Source: CAD feature listing. Evaluate the final solid. Frame: model axes, mm. Face numbers are marked on the shaded views. A direction names the side the tool comes from. Coordinates: 2 decimals unless noted, no trailing zeros. Loops run counter-clockwise (first coordinate to the right, second up) from the corner with the lowest first, then second, coordinate; pieces in that order, holes last. Notation, with made-up numbers: (-37.5, 0) -> (-3.5, 0) arc R9 ccw to (-3.5, 10) -> close; hole circle Ø1 at (-10, 31). An arc over 180 degrees is marked (long way). Answer as CSV lines item,"result".
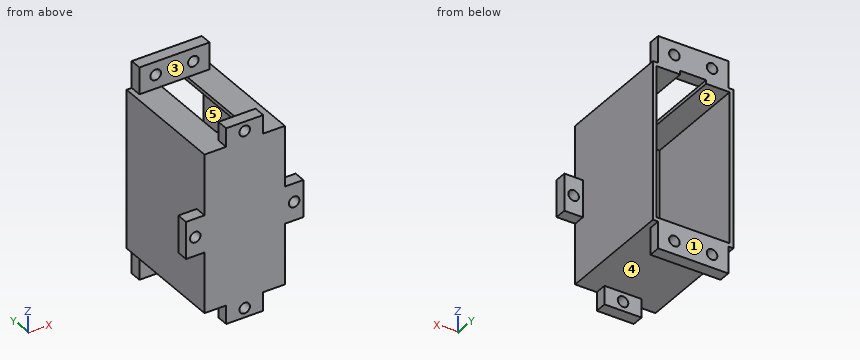
from build123d import *

# Parameters (mm, degrees)
SKETCH1_R           = 1.425
BOSS_EXTRUDE1_DEPTH = 3.175
SKETCH2_W           = 21.685
SKETCH2_H           = 42.7
SKETCH2_W_2         = 19.685
SKETCH2_H_2         = 40.7
BOSS_EXTRUDE2_DEPTH = 28.905
SKETCH3_W           = 18.923
SKETCH3_H           = 7.239
SKETCH3_R           = 1.425
BOSS_EXTRUDE3_DEPTH = 3.175
SKETCH4_W           = 7
SKETCH4_H           = 25.77275476
CUT_EXTRUDE1_DEPTH  = 3.175


with BuildPart() as part:
    # Sketch1 → Boss-Extrude1 (new body)
    with BuildSketch(Plane(origin=(0, 0, 0), x_dir=(1, 0, 0), z_dir=(0, 1, 0))):
        Polygon((10.8425, -21.35), (5, -21.35), (5, -26.35), (-5, -26.35), (-5, -21.35), (-10.8425, -21.35), (-10.8425, -5), (-15.8425, -5), (-15.8425, 5), (-10.8425, 5), (-10.8425, 21.35), (-5, 21.35), (-5, 26.35), (5, 26.35), (5, 21.35), (10.8425, 21.35), (10.8425, 5), (15.8425, 5), (15.8425, -5), (10.8425, -5), align=None)
        with Locations(Location((0, 23.85, 0), (0, 0, 270))):
            Circle(SKETCH1_R, mode=Mode.SUBTRACT)
        with Locations(Location((-13.3425, 0, 0), (0, 0, 270))):
            Circle(SKETCH1_R, mode=Mode.SUBTRACT)
        with Locations(Location((13.3425, 0, 0), (0, 0, 270))):
            Circle(SKETCH1_R, mode=Mode.SUBTRACT)
        with Locations(Location((0, -23.85, 0), (0, 0, 270))):
            Circle(SKETCH1_R, mode=Mode.SUBTRACT)
    extrude(amount=BOSS_EXTRUDE1_DEPTH)

    # Sketch2 → Boss-Extrude2 (add)
    with BuildSketch(Plane(origin=(0, 3.175, 0), x_dir=(1, 0, 0), z_dir=(0, 1, 0))):
        Rectangle(SKETCH2_W, SKETCH2_H)
        Rectangle(SKETCH2_W_2, SKETCH2_H_2, mode=Mode.SUBTRACT)
    extrude(amount=BOSS_EXTRUDE2_DEPTH)

    # Sketch3 → Boss-Extrude3 (add)
    # profile 1 of 2: a face of its own
    with BuildSketch(Plane(origin=(0, 32.08, 0), x_dir=(1, 0, 0), z_dir=(0, 1, 0))):
        with Locations((0, 24.9695)):
            Rectangle(SKETCH3_W, SKETCH3_H)
        with Locations(Location((-5.08, 25.049, 0), (0, 0, 270))):
            Circle(SKETCH3_R, mode=Mode.SUBTRACT)
        with Locations(Location((5.08, 25.049, 0), (0, 0, 270))):
            Circle(SKETCH3_R, mode=Mode.SUBTRACT)
    # profile 2 of 2: a face of its own
    with BuildSketch(Plane(origin=(0, 32.08, 0), x_dir=(1, 0, 0), z_dir=(0, 1, 0))):
        with Locations((0, -24.9695)):
            Rectangle(SKETCH3_W, SKETCH3_H)
        with Locations(Location((-5.08, -25.049, 0), (0, 0, 270))):
            Circle(SKETCH3_R, mode=Mode.SUBTRACT)
        with Locations(Location((5.08, -25.049, 0), (0, 0, 270))):
            Circle(SKETCH3_R, mode=Mode.SUBTRACT)
    extrude(amount=-BOSS_EXTRUDE3_DEPTH)

    # Sketch4 → Cut-Extrude1 (cut)
    with BuildSketch(Plane.XY.offset(21.35)):
        with Locations((0, 19.19362262)):
            Rectangle(SKETCH4_W, SKETCH4_H)
    extrude(amount=-CUT_EXTRUDE1_DEPTH, mode=Mode.SUBTRACT)


solid = part.part
(1) Cut plane C-C (x = 0). Return the cut outline in (y, z) (3 decimals), then the cut area to 3 significant figures.
Computed values:
outline,"(0, -26.35) -> (3.175, -26.35) -> (3.175, -25.275) -> (0, -25.275) -> close; (0, -22.425) -> (3.175, -22.425) -> (3.175, -21.35) -> (28.905, -21.35) -> (28.905, -28.589) -> (32.08, -28.589) -> (32.08, -20.35) -> (3.175, -20.35) -> (3.175, 20.35) -> (6.307, 20.35) -> (6.307, 21.35) -> (3.175, 21.35) -> (3.175, 22.425) -> (0, 22.425) -> close; (0, 25.275) -> (3.175, 25.275) -> (3.175, 26.35) -> (0, 26.35) -> close; (28.905, 21.35) -> (32.08, 21.35) -> (32.08, 28.589) -> (28.905, 28.589) -> close"
area,"227 mm^2"
(2) Access query for the marked faces 1, 2 and 3. Directions: +Z, -Z, +X, -X, +Y, -Y. A direction counts if a zero-diameter tool reaches every point of the face in a straight line with its end or side. Return the directions, or none.
Computed values:
face 1,"+Z, -Z, +X, -X, +Y"
face 2,"+Y"
face 3,"+Z, +X, -X"
(3) Cut plane A-A (y = 4). Return the cut outline in (x, z).
Computed values:
outline,"(-10.84, -21.35) -> (10.84, -21.35) -> (10.84, 21.35) -> (-10.84, 21.35) -> close; hole (-9.84, -20.35) -> (9.84, -20.35) -> (9.84, 20.35) -> (-9.84, 20.35) -> close"
(4) Material intervals for L1, parallel to Z at x = 5, y = 29; L2, parallel to Z at x = 5, y = 18; L3, parallel to X at y = 17.5, z = 13.5, sorted ascending. Write a range as [from, to].
Computed values:
L1,"[-28.59, -26.47], [-23.63, -20.35], [20.35, 23.63], [26.47, 28.59]"
L2,"[-21.35, -20.35], [20.35, 21.35]"
L3,"[-10.84, -9.84], [9.84, 10.84]"
(5) Cut plane D-D (z = 6). Return the cut outline in (x, y) (1 decimal), then the cut area to 3 significant figures.
Computed values:
outline,"(-10.8, 0) -> (10.8, 0) -> (10.8, 32.1) -> (9.8, 32.1) -> (9.8, 3.2) -> (-9.8, 3.2) -> (-9.8, 32.1) -> (-10.8, 32.1) -> close"
area,"127 mm^2"
(6) Pin query (flat end, axial travel): pin 1 Ø1 at (x, z) = (8.5, 9) entering from -Y; pin 2 Ø3 at (x, y) = (12, 20) entering from -Z; pin 3 Ø1 at (y, z) = (1, -22.5) entering from -X; pin 4 Ø1.5 at (y, z) = (21.5, -3) entering from -X. Return the tip coordinate at first contact, or that it passes through.
Computed values:
pin 1,"y = 0"
pin 2,"z = -21.35"
pin 3,"x = -5"
pin 4,"x = -10.84"
(7) Draft query along X for the marked faces 4 and 5. Return one class per face: released by +X, released by -X, zero draft, split by the parting line, or undercut.
Computed values:
face 4,"zero draft"
face 5,"undercut"
(8) Cut plane B-B (z = 0). Return the cut outline in (x, y) (1 decimal).
Computed values:
outline,"(-15.8, 0) -> (-14.8, 0) -> (-14.8, 3.2) -> (-15.8, 3.2) -> close; (-11.9, 0) -> (11.9, 0) -> (11.9, 3.2) -> (10.8, 3.2) -> (10.8, 32.1) -> (9.8, 32.1) -> (9.8, 3.2) -> (-9.8, 3.2) -> (-9.8, 32.1) -> (-10.8, 32.1) -> (-10.8, 3.2) -> (-11.9, 3.2) -> close; (14.8, 0) -> (15.8, 0) -> (15.8, 3.2) -> (14.8, 3.2) -> close"
